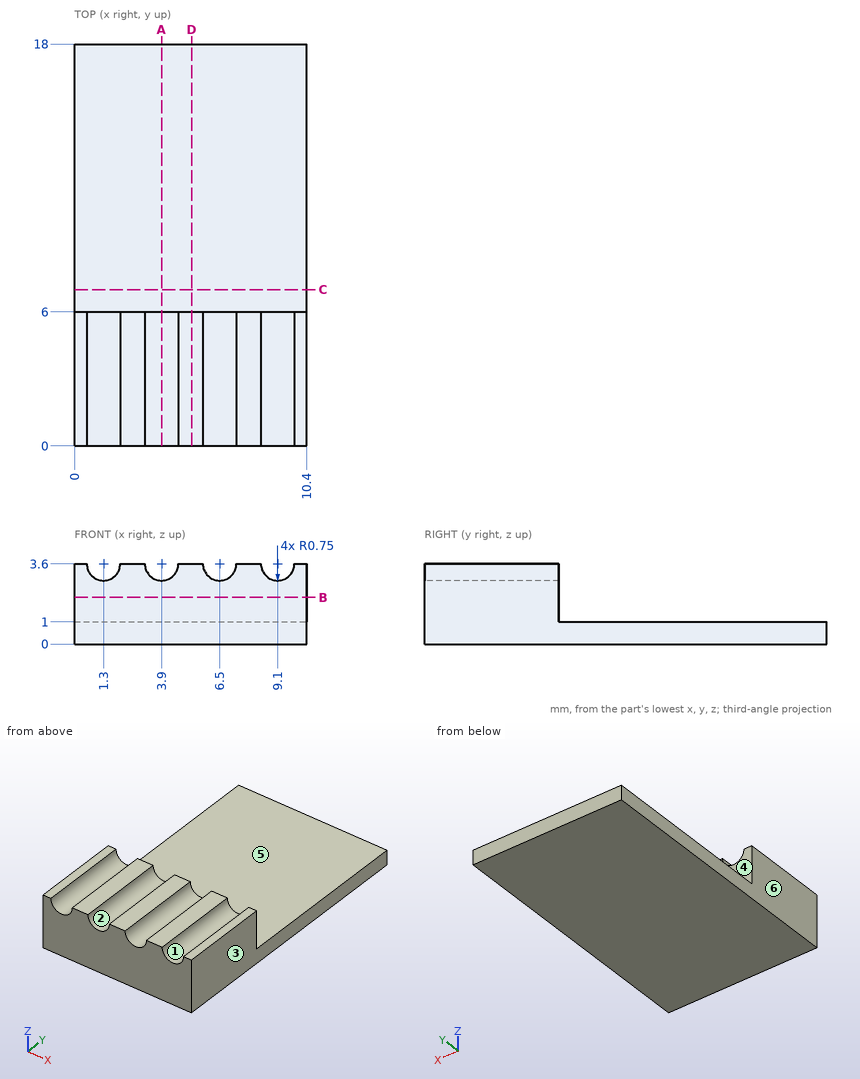
For this review, use the dimensioned drawing (mm, ordinates from the lowest corner) and the shaded views. A direction names the side the tool comes from. Give positions to 0.01 mm unless a question says otherwise; leave off trailing zeros. Write each loop counter-clockwise with the first axis right and the second up, starting at its lowest first coordinate (ties: lowest second). Pieces come first, ordered by that corner, then holes. Notation, with made-up numbers: M -15.5,45 L -4.5,45 A17 cw -4.5,75 Z; hole C 22.25,0.25 d11. An arc over 180 degrees is marked long. Write item = value, one per line. Start each with the question number.
Q1. We need section D-D (x = 5.25). State the section outline as (y, z) points, plus the area to 3 significant figures.
Q2. For line 1 (Y direction, x = 3.75, z = 1.9); line 2 (Z direction, x = 6.25, y = 8.75); line 3 (Z direction, x = 4.5, y = 2.5), list the stretches that pass through material, from the lowest coordinate up.
Q3. Mouldability with a two-part tool opening along X and no side actions: class the marked faces 1, 2, 3 and 4 as released by +X, released by -X, zero draft, split by the parting line, or undercut.
Q4. We need section C-C (y = 7). State the section outline as (x, z) points, plus the area to 3 significant figures.
Q5. We need section A-A (x = 3.9). State the section outline as (y, z) points, plus the area to 3 significant figures.
Q6. We need section B-B (z = 2.1). State the section outline as (x, y) points.
Q7. Machinability: for the marked faces 5 and 6, which of the approach directions +Z, -Z, +X, -X, +Y, -Y give a long, thin tool a straight path to every point of the face, cutting with its end or side? Answer none if there is none.
Q8. Clearance check with a flat-ended pin moving along its axis: pin 1 (5 mm diameter, centred on x = 8.5, y = 16, fed in from -Z). State where the tip first meets the part, or that it passes through.
Result set:
q1.outline = M 0,0 L 18,0 L 18,1 L 6,1 L 6,3.6 L 0,3.6 Z
q1.area = 33.6 mm2
q2.line_1 = 0 to 6
q2.line_2 = 0 to 1
q2.line_3 = 0 to 3.15
q3.face_1 = undercut
q3.face_2 = undercut
q3.face_3 = released by +X
q3.face_4 = zero draft
q4.outline = M 0,0 L 10.4,0 L 10.4,1 L 0,1 Z
q4.area = 10.4 mm2
q5.outline = M 0,0 L 18,0 L 18,1 L 6,1 L 6,2.85 L 0,2.85 Z
q5.area = 29.1 mm2
q6.outline = M 0,0 L 10.4,0 L 10.4,6 L 0,6 Z
q7.face_5 = +Z, +X, -X, +Y
q7.face_6 = +Z, -Z, -X, +Y, -Y
q8.pin_1 = 0
